Source: CAD feature listing. Evaluate the final solid. Frame: model axes, mm. Face numbers are marked on the shaded views. A direction names the side the tool comes from. Give positions to 0.01 mm unless a question says otherwise; leave off trailing zeros. Order: outer loops, then holes, each group sorted by start corner. A loop starts at its lowest first (then second) coordinate and runs counter-clockwise, first axis right, second up.
from build123d import *

# Parameters (mm, degrees)
F0_W     = 838.2
F0_H     = 508
F0_W_2   = 685.8
F0_H_2   = 355.6
F1_DEPTH = 228.6
F2_T     = -0.254
F4_DEPTH = 838.2


with BuildPart() as f1:
    # F0 (on Top) → F1 (new body)
    with BuildSketch(Plane.XY):
        with Locations((-259.4876274824, 118.1668707132)):
            Rectangle(F0_W, F0_H)
        with Locations((-259.4876274824, 118.1668707132)):
            Rectangle(F0_W_2, F0_H_2, mode=Mode.SUBTRACT)
        with Locations((-259.4876274824, 118.1668707132)):
            Rectangle(F0_W_2, F0_H_2)
    extrude(amount=F1_DEPTH)

    # F2
    f2_openings = [f1.faces().sort_by_distance(p)[0] for p in [
        (-259.487627, 118.166871, 0),
    ]]
    offset(amount=F2_T, openings=f2_openings)

    # F3 (on face) → F4 (join)
    with BuildSketch(Plane.YZ.offset(159.6123725176)):
        Polygon((118.1668707132, 279.4), (-135.8331292868, 228.6), (118.1668707132, 228.6), align=None)
        Polygon((118.1668707132, 279.4), (118.1668707132, 228.6), (372.1668707132, 228.6), align=None)
    extrude(amount=-F4_DEPTH)


solid = f1.part
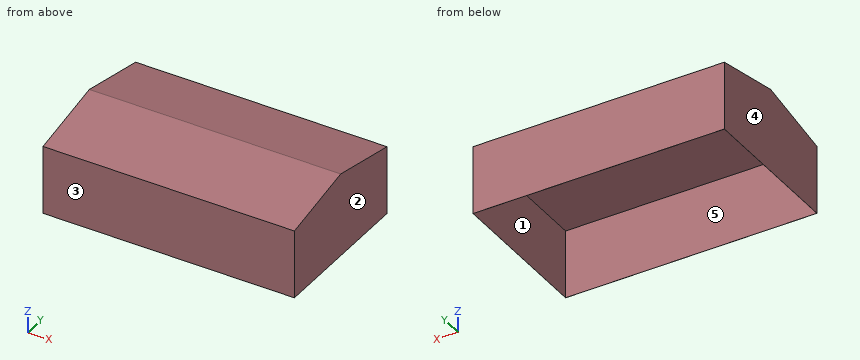
1) Pull-direction query (Y, two-part tool) for the marked faces 3, 4 and 5; classes: +Y half, -Y half, draft (parallel to the pull), parting line (faces both ways), or undercut.
Checks:
face 3: -Y half
face 4: draft
face 5: undercut
2) Ray query, L1, parallel to Y at x = -37, z = 98; L2, parallel to X at y = 304.5, z = 145; L3, parallel to Z at x = -480, y = 299.5. Return the intervals inside material, ascending.
Checks:
L1: y = -135.83 to -135.58, 371.91 to 372.17
L2: x = -678.59 to -678.33, 159.36 to 159.61
L3: z = 228.35 to 243.13
3) Section query A-A on z = 208. Output: boundary loops of the cut face in (x, y), and give its area (3 significant figures).
Checks:
outline: (-678.59, -135.83) - (159.61, -135.83) - (159.61, 372.17) - (-678.59, 372.17) - close; hole (-678.33, -135.58) - (159.36, -135.58) - (159.36, 371.91) - (-678.33, 371.91) - close
area: 684 mm2
4) Section query D-D on y = 329. Output: boundary loops of the cut face in (x, z).
Checks:
outline: (-678.59, 0) - (-678.33, 0) - (-678.33, 228.35) - (159.36, 228.35) - (159.36, 0) - (159.61, 0) - (159.61, 237.23) - (-678.59, 237.23) - close
5) Reachability of the marked faces 1 and 2 from +Z, -Z, +X, -X, +Y, -Y: full face, straight path, thin tool, end or side. Return the list, or none.
Checks:
face 1: -Z
face 2: +Z, -Z, +X, +Y, -Y
6) First-contact query: pin 1 Ø1 at (x, y) = (-154, 165.5) entering from -Z. Flat tip, straight axial feed; report the tip coordinate or a pass-through.
Checks:
pin 1: stops at z = 228.35
7) Section query B-B on x = 74.5. Output: boundary loops of the cut face in (y, z), and give its area (3 significant figures).
Checks:
outline: (-135.83, 0) - (-135.58, 0) - (-135.58, 228.35) - (371.91, 228.35) - (371.91, 0) - (372.17, 0) - (372.17, 228.6) - (118.17, 279.4) - (-135.83, 228.6) - close
area: 13,100 mm2
8) Section query C-C on y = 41. Output: boundary loops of the cut face in (x, z).
Checks:
outline: (-678.59, 0) - (-678.33, 0) - (-678.33, 228.35) - (159.36, 228.35) - (159.36, 0) - (159.61, 0) - (159.61, 263.97) - (-678.59, 263.97) - close
